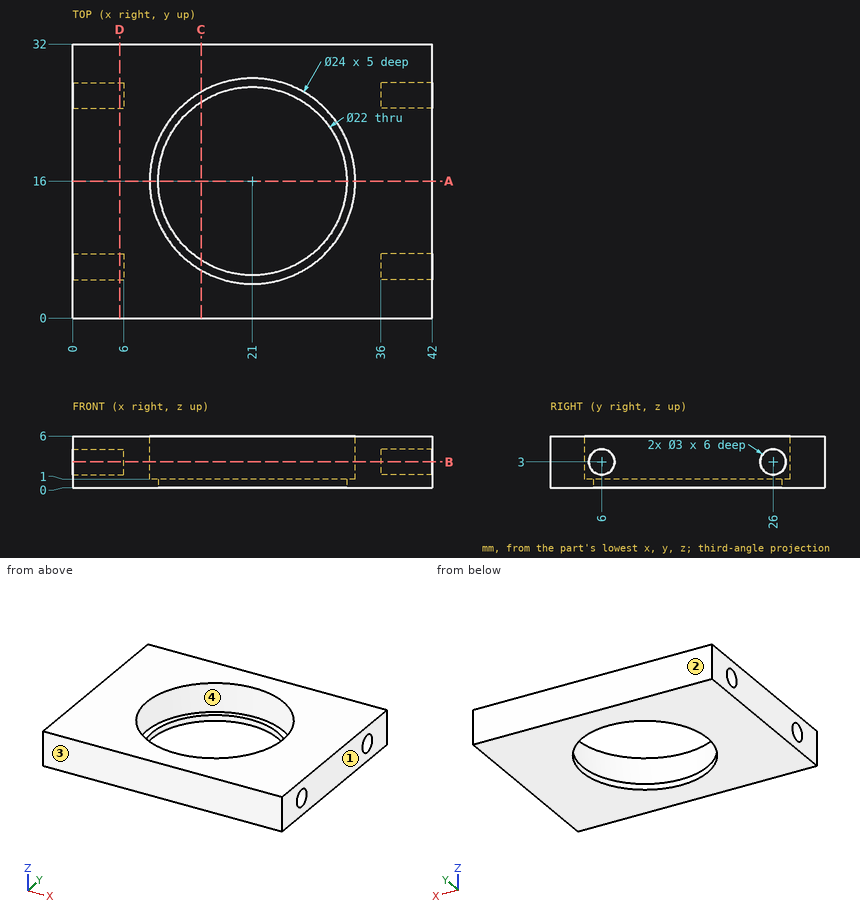
Could you check a few things on this drawing? It's one solid part, dimensions in mm from its lowest x, y, z. Give positions to 0.01 mm unless a question says otherwise; leave off trailing zeros. Order: outer loops, then holes, each group sorted by start corner. A loop starts at its lowest first (then second) coordinate and runs counter-clockwise, first axis right, second up. Notation, with made-up numbers: (87.25, 9.5) - (125.25, 9.5) arc R18 cw to (125.25, 13.5) - close; hole circle Ø8 at (32.25, 76). An arc over 180 degrees is marked (long way). One line per question, with ' | ' between items. Start each with the question number.
Item 1: I want a section at B-B on z = 3. Write out the boundary of the cut face in (x, y).
Item 2: I want a section at D-D on x = 5.5. Write out the boundary of the cut face in (y, z).
Item 3: Thinking about a two-plate mould opening in Y: for the marked faces 1, 2, 3 and 4, which applies, pulls with the +Y half, pulls with the -Y half, needs draft (parallel to the pull), parting line crosses it, or undercut?
Item 4: I need wall thicknesses on probe 1 along Y at (x, z) = (21, 3.65); probe 2 along Y at (x, z) = (21, 0.3); probe 3 along X at (y, z) = (15, 0.4). Which ranges of each line are inside material? Lowest first, please. Write a range as [from, to].
Item 5: I want a section at C-C on x = 15. Write out the boundary of the cut face in (y, z).
Item 6: I want a section at A-A on y = 16. Write out the boundary of the cut face in (x, z), then the cut area to 3 significant figures.
Item 7: I'm going to push flat-ended pins straight in: pin 1 Ø2.5 at (y, z) = (6, 3) entering from +X; pin 2 Ø14.5 at (x, y) = (21, 16) entering from +Z; pin 3 Ø0.9 at (y, z) = (6.5, 3.5) entering from -X. Where does each tip first touch, or does it pass through?
Verdict:
1) outline: (0, 0) - (42, 0) - (42, 4.5) - (36, 4.5) - (36, 7.5) - (42, 7.5) - (42, 24.5) - (36, 24.5) - (36, 27.5) - (42, 27.5) - (42, 32) - (0, 32) - (0, 27.5) - (6, 27.5) - (6, 24.5) - (0, 24.5) - (0, 7.5) - (6, 7.5) - (6, 4.5) - (0, 4.5) - close; hole circle Ø24 at (21, 16)
2) outline: (0, 0) - (32, 0) - (32, 6) - (0, 6) - close; hole circle Ø3 at (6, 3); hole circle Ø3 at (26, 3)
3) face 1: needs draft | face 2: pulls with the +Y half | face 3: pulls with the -Y half | face 4: undercut
4) probe 1: [0, 4], [28, 32] | probe 2: [0, 5], [27, 32] | probe 3: [0, 10.05], [31.95, 42]
5) outline: (0, 0) - (6.78, 0) - (6.78, 1) - (5.61, 1) - (5.61, 6) - (0, 6) - close; (25.22, 0) - (32, 0) - (32, 6) - (26.39, 6) - (26.39, 1) - (25.22, 1) - close
6) outline: (0, 0) - (10, 0) - (10, 1) - (9, 1) - (9, 6) - (0, 6) - close; (32, 0) - (42, 0) - (42, 6) - (33, 6) - (33, 1) - (32, 1) - close | area: 110 mm^2
7) pin 1: x = 36 | pin 2: through | pin 3: x = 6
